Can you work these out from the drawing? Everything is in mm from the part's minimum corner. Round coordinates to 2 decimals unless told otherwise and drop trailing zeros. Write each loop counter-clockwise with the first axis right and the second up, starting at its lowest first coordinate (ties: lowest second). Pieces come first, ordered by that corner, then holes. Notation, with made-up numbers: M 70.25,87 L 115.25,87 A14 ccw 115.25,102 Z; hole C -27,-13.75 d9. An arc over 180 degrees is marked long. Answer in a Markdown table with one row per item. Add a question column.
(1) If I drill on probe 1 along Z at (x, y) = (28, 5.25); probe 2 along Y at (x, z) = (19.5, 34); probe 3 along Y at (x, z) = (29, 43.5), over which ranges is the centre line in solid material (lowest first)?
(2) I'm going to push a flat-ended pin straight in: pin 1 (6 mm diameter, centred on x = 8.5, y = 7.5, fed in from -Z). Where does the tip first touch, or does it pass through?
(3) If we mould it in two halves opening along Z, with no side actions, what happens to the marked faces 1, 2, 3 and 4? For each: released by +Z, released by -Z, zero draft, split by the parting line, or undercut.
(4) Suppose I cut it at C-C, the plane x = 21. Write out the boundary of the cut face in (y, z), then the cut area to 3 significant figures.
(5) Suppose I cut it at B-B, the plane z = 27. Write out the boundary of the cut face in (x, y).
(6) Suppose I cut it at A-A, the plane y = 7. Write out the boundary of the cut face in (x, z), then the cut area to 3 significant figures.
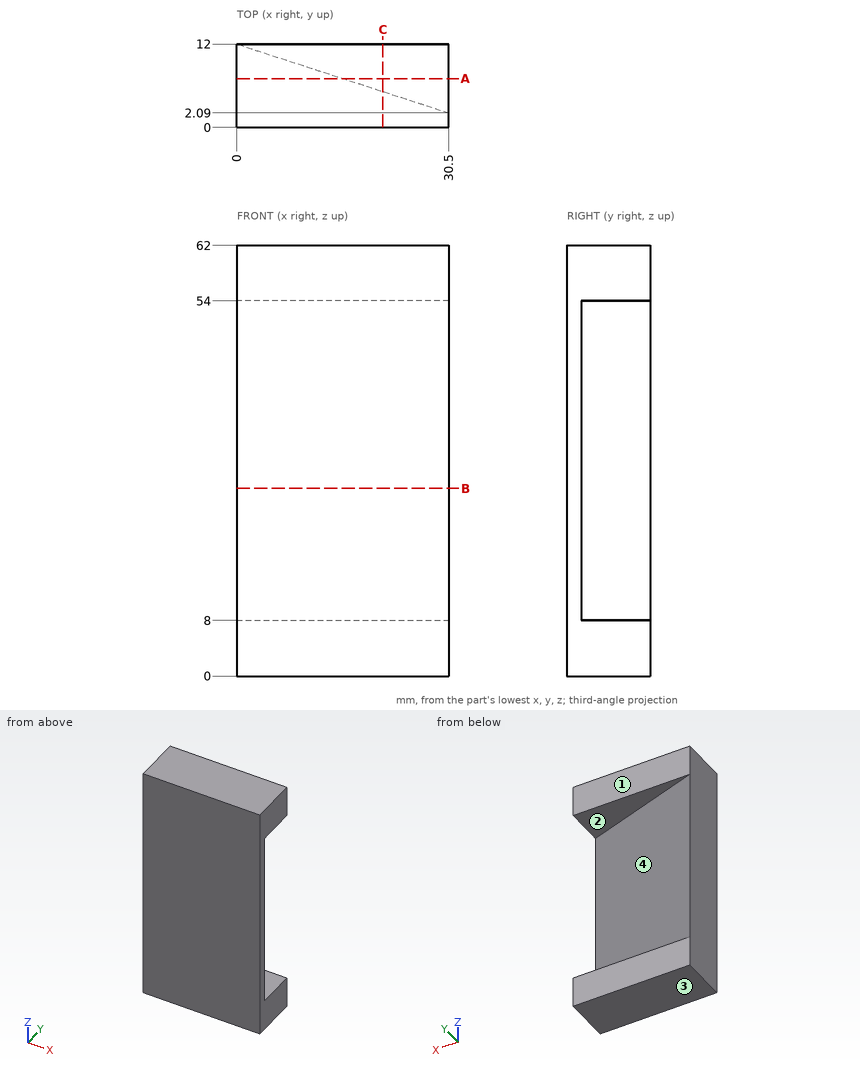
Calculated:
| question | item | result |
|---|---|---|
| 1 | probe 1 | 0 to 8, 54 to 62 |
| 1 | probe 2 | 0 to 5.66 |
| 1 | probe 3 | 0 to 2.58 |
| 2 | pin 1 | z = 0 |
| 3 | face 1 | zero draft |
| 3 | face 2 | undercut |
| 3 | face 3 | released by -Z |
| 3 | face 4 | undercut |
| 4 | outline | M 0,0 L 12,0 L 12,8 L 5.18,8 L 5.18,54 L 12,54 L 12,62 L 0,62 Z |
| 4 | area | 430 mm² |
| 5 | outline | M 0,0 L 30.5,0 L 30.5,2.09 L 0,12 Z |
| 6 | outline | M 0,0 L 30.5,0 L 30.5,8 L 15.39,8 L 15.39,54 L 30.5,54 L 30.5,62 L 0,62 Z |
| 6 | area | 1,200 mm² |
